Autodesk Inventor part; units mm, degrees
ref_plane "YZ Plane" through (0, 0, 0) normal (1, 0, 0) x (0, 1, 0)
ref_plane "XZ Plane" through (0, 0, 0) normal (0, 1, 0) x (-1, 0, 0)
ref_plane "XY Plane" through (0, 0, 0) normal (0, 0, 1) x (1, 0, 0)
sketch "Sketch1" plane through (0, 0, 0) normal (0, 1, 0) x (-1, 0, 0)
  circle A0 centre (0, 0) radius 3
  dimension "d0" = 6
extrude "Extrusion1" add sketch "Sketch1" along normal blind 12
thread "Thread1"
chamfer "Chamfer1" distance 0.5 angle 45 1 edges at (3, 0, 0)
sketch "Sketch2" plane through (0, 12, 0) normal (0, 1, 0) x (1, 0, 0)
  circle A0 centre (0, 0) radius 5
  dimension "d8" = 10
extrude "Extrusion2" add sketch "Sketch2" along normal blind 6
sketch "Sketch3" plane through (0, 18, 0) normal (0, 1, 0) x (1, 0, 0)
  line L0 (-3.4231, 1.9737) -> (-0.0023, 3.9513)
  line L1 (-0.0023, 3.9513) -> (3.4208, 1.9776)
  line L2 (3.4208, 1.9776) -> (3.4231, -1.9737)
  line L3 (3.4231, -1.9737) -> (0.0023, -3.9513)
  line L4 (0.0023, -3.9513) -> (-3.4208, -1.9776)
  line L5 (-3.4208, -1.9776) -> (-3.4231, 1.9737)
  point P0 (0, 0)
  point P1 (0, 0)
extrude "Extrusion3" cut sketch "Sketch3" against normal blind 4
properties part number "M6_12mm" material "Steel, Carbon"
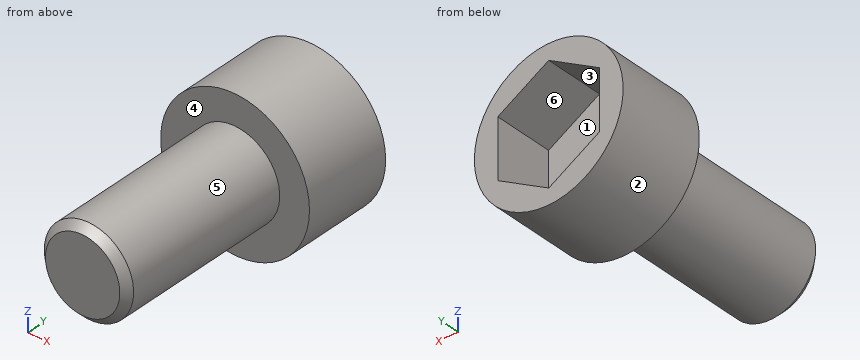
Check sheet for the modelled part. Datum: model origin and axes. Units: mm. Face numbers are marked on the shaded views. A direction names the side the tool comes from. Round coordinates to 2 decimals unless told otherwise and drop trailing zeros. Order: outer loops, then holes, each group sorted by start corner. A loop starts at its lowest first (then second) coordinate and runs counter-clockwise, first axis right, second up. Notation, with made-up numbers: M 88,-38 L 128,-38 A25 cw 128,-9 Z; hole C -15.75,50.5 d6. An arc over 180 degrees is marked long. One line per item, written item: value. Start each with the question number.
1. Release check for a two-part mould opening along Z. For the marked faces 3, 4, 5 and 6 record: released by +Z, released by -Z, zero draft, split by the parting line, or undercut.
2. Section check C-C on y = 8.25. Enter the section's corners in (x, z), and give its area (3 significant figures).
3. Section check D-D on x = 4.5. Enter the section's corners in (y, z).
4. Access from +Z, -Z, +X, -X, +Y, -Y to the whole of each face (thin tool, end or side, straight path). Record for the marked faces 1 and 2.
5. Gauge pin test, flat ends, axial feed: P1, Ø5, axis at x = -3.5, y = 5.5, coming from the -Z side; P2, Ø4, axis at x = -3.5, y = 5, coming from the -Z side. Record the tip position at first contact, or that the pin passes through.
6. Scan lines: line 1 along Y through (x, z) = (-0.25, 3.5); line 2 along Y through (x, z) = (-2.75, -3.5); line 3 along Z through (x, y) = (0, 11.75). Record each from-to range of solid material in increasing order.
7. Section check A-A on z = 0. Enter the section's corners in (x, y).
8. Section check B-B on x = -4. Enter the section's corners in (y, z), and give its area (3 significant figures).
Results found:
1. face 3: undercut
1. face 4: zero draft
1. face 5: split by the parting line
1. face 6: undercut
2. outline: C 0,0 d6
2. area: 28.3 mm^2
3. outline: M 12,-2.18 L 18,-2.18 L 18,2.18 L 12,2.18 Z
4. face 1: +Y
4. face 2: +Y, -Y
5. P1: z = -2.83
5. P2: z = -2.6
6. line 1: 12 to 14
6. line 2: 12 to 18
6. line 3: -3 to 3
7. outline: M -5,12 L -3,12 L -3,0.5 L -2.5,0 L 2.5,0 L 3,0.5 L 3,12 L 5,12 L 5,18 L 3.42,18 L 3.42,14 L -3.42,14 L -3.42,18 L -5,18 Z
8. outline: M 12,-3 L 18,-3 L 18,3 L 12,3 Z
8. area: 36.0 mm^2
